The listing builds one solid part. Answer for the finished solid, in the listing's coordinates (mm). Face numbers are marked on the shaded views. Give positions to 0.01 mm unless a question says otherwise; leave off trailing zeros. Order: outer loops, then holes, each group sorted by start corner. A loop starts at its lowest first (then second) coordinate and runs counter-clockwise, first axis right, second up.
Autodesk Inventor part; units mm, degrees
ref_plane "YZ Plane" through (0, 0, 0) normal (1, 0, 0) x (0, 1, 0)
ref_plane "XZ Plane" through (0, 0, 0) normal (0, 1, 0) x (-1, 0, 0)
ref_plane "XY Plane" through (0, 0, 0) normal (0, 0, 1) x (1, 0, 0)
sketch "Sketch1" plane through (0, 0, 0) normal (0, 1, 0) x (-1, 0, 0)
  line L0 (8.4018, 18.0616) -> (-10.6482, 18.0616)
  line L1 (-10.6482, 18.0616) -> (-10.6482, -29.5634)
  line L2 (-10.6482, -29.5634) -> (8.4018, -29.5634)
  line L3 (8.4018, -29.5634) -> (8.4018, 18.0616)
  circle A0 centre (-1.1232, -5.7509) radius 4.0005
  point P0 (0, 0)
  dimension "d0" = 19.05
  dimension "d1" = 47.625
  dimension "d2" = 8.001
extrude "Extrusion1" add sketch "Sketch1" along normal blind 12.7
sketch "Sketch2" plane through (-8.4018, 0, 18.0616) normal (0, 0, 1) x (1, 0, 0)
  line L0 (0, 0) -> (0, 12.7)
  line L1 (0, 6.35) -> (18.844, 6.35)
  circle A0 centre (3.175, 6.35) radius 0.889
  circle A1 centre (15.875, 6.35) radius 0.889
  point P0 (8.4018, 0)
  dimension "d5" = 12.7
  dimension "d6" = 3.175
  dimension "d7" = 1.778
  dimension "d8" = 1.778
extrude "Extrusion2" cut sketch "Sketch2" against normal blind 12.7
sketch "Sketch3" plane through (10.6482, 0, -29.5634) normal (0, 0, -1) x (-1, 0, 0)
  circle A0 centre (3.175, 6.35) radius 0.889
  circle A1 centre (15.875, 6.35) radius 0.889
  point P0 (10.6482, 0)
extrude "Extrusion3" cut sketch "Sketch3" against normal blind 12.7
chamfer "Chamfer1" distance 3.175 angle 45 4 edges at (10.6482, 12.7, -5.7509) (-8.4018, 12.7, -5.7509) (1.1232, 12.7, 18.0616) (1.1232, 12.7, -29.5634)
sketch "Sketch4" plane through (0, 12.7, 0) normal (0, 1, 0) x (1, 0, 0)
  circle A0 centre (1.1232, 5.7509) radius 4.0005
  line L0 (2.2662, 1.7504) -> (2.2662, -0.7896)
  line L1 (2.2662, -0.7896) -> (-0.0198, -0.7896)
  line L2 (-0.0198, -0.7896) -> (-0.0198, 1.7504)
  line L3 (-0.0198, 1.7504) -> (-0.0198, 1.9172)
  line L4 (2.2662, 1.7504) -> (2.2662, 1.9172)
  line L5 (2.2662, 12.2914) -> (2.2662, 9.7514)
  line L6 (-0.0198, 12.2914) -> (2.2662, 12.2914)
  line L7 (-0.0198, 9.7514) -> (-0.0198, 12.2914)
  line L8 (2.2662, 9.7514) -> (2.2662, 9.5847)
  line L9 (-6.1158, 16.8634) -> (-4.3378, 16.8634)
  line L10 (-0.0198, 9.7514) -> (-0.0198, 9.5847)
  point P0 (0, 0)
  point P1 (1.1232, 1.7504)
  dimension "d18" = 2.54
  dimension "d21" = 360
extrude "Extrusion4" cut sketch "Sketch4" against normal blind 2.54 contours A0 L10 L7 L6 L5 L8 | L4 L0 L1 L2 L3 A0
properties part number "bottom_anchor"
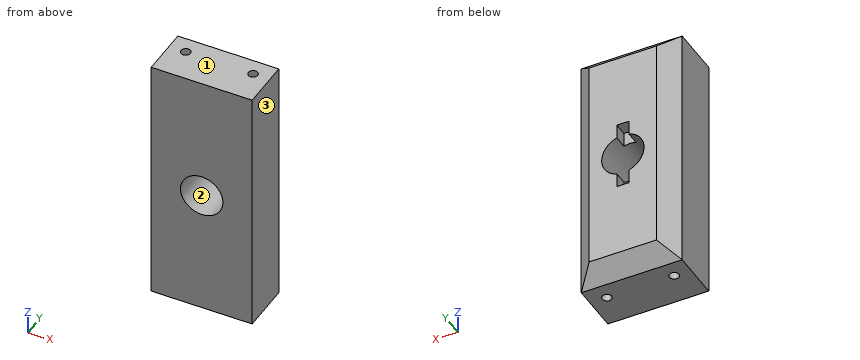
1) Find section C-C (z = -8). Write down the section's boundary in (x, y) (3 decimals), then the cut area to 3 significant figures.
Geometry says:
outline: (-8.402, 0) - (-2.185, 0) - (-2.185, 12.7) - (-5.227, 12.7) - (-8.402, 9.525) - close; (4.432, 0) - (10.648, 0) - (10.648, 9.525) - (7.473, 12.7) - (4.432, 12.7) - close
area: 148 mm2
2) For a pull along Z with two mould halves and no side action, classify the marked faces 1, 2 and 3 as +Z half, -Z half, draft (parallel to the pull), parting line (faces both ways), or undercut.
Geometry says:
face 1: +Z half
face 2: undercut
face 3: draft
3) Find section B-B (y = 11). Write down the section's boundary in (x, z).
Geometry says:
outline: (-6.93, -28.09) - (9.17, -28.09) - (9.17, 16.59) - (-6.93, 16.59) - close; hole (-0.02, -12.29) - (2.27, -12.29) - (2.27, -9.58) arc R4 ccw to (2.27, -1.92) - (2.27, 0.79) - (-0.02, 0.79) - (-0.02, -1.92) arc R4 ccw to (-0.02, -9.58) - close
4) Find section A-A (x = 1.75). Write down the section's boundary in (y, z) (3 decimals), then the cut area to 3 significant figures.
Geometry says:
outline: (0, -29.563) - (9.525, -29.563) - (12.7, -26.388) - (12.7, -12.291) - (10.16, -12.291) - (10.16, -9.702) - (0, -9.702) - close; (0, -1.8) - (10.16, -1.8) - (10.16, 0.79) - (12.7, 0.79) - (12.7, 14.887) - (9.525, 18.062) - (0, 18.062) - close
area: 481 mm2
5) Find section D-D (z = 3). Write down the section's boundary in (x, y) (3 decimals), then the cut area to 3 significant figures.
Geometry says:
outline: (-8.402, 0) - (10.648, 0) - (10.648, 9.525) - (7.473, 12.7) - (-5.227, 12.7) - (-8.402, 9.525) - close
area: 232 mm2
6) Straight lines are drawn through the part: probe 1 along X at (y, z) = (6.35, 11.5); probe 2 along X at (y, z) = (11.5, -7.5); probe 3 along Y at (x, z) = (-5.75, -19). For each, find the intervals that lie inside material, in ascending order.
Geometry says:
probe 1: x = -8.4 to -6.12, -4.34 to 6.58, 8.36 to 10.65
probe 2: x = -6.43 to -2.47, 4.72 to 8.67
probe 3: y = 0 to 5.63, 7.07 to 12.18
7) Given P1, Ø0.8, axis at y = 12, z = -10.5, coming from the -X side; P2, Ø0.9, axis at x = 7.5, y = 6.5, coming from the +Z side; P3, Ø0.7, axis at x = 1.5, y = 11, coming from the -Z side; P4, Ø5, axis at x = 1.12, z = -5.75, coming from the +Y side, each flat-ended and moving along its own axis, determine where each tip first touches the part or whether it passes through.
Geometry says:
P1: stops at x = -6.33
P2: stops at z = 5.36
P3: stops at z = -28.44
P4: passes through
